```python
from build123d import *

# Parameters (mm, degrees)
EXTRUDE_1_DEPTH        = 35
SKETCH_4_W             = 142
SKETCH_4_H             = 75
CUT_EXTRUDE_2_DEPTH    = 25
SKETCH_5_R             = 29
CUT_EXTRUDE_3_DEPTH    = 11
CHAMFER_3_SIZE         = 3
FILLET_2_R             = 3
SKETCH_7_R             = 3.2
SKETCH_7_R_2           = 3.25
CUT_EXTRUDE_4_DEPTH    = 11
SKETCH_8_R             = 25.025
CUT_EXTRUDE_5_DEPTH    = 11
SKETCH_9_R             = 5.25
CUT_EXTRUDE_6_DEPTH    = 25
HOLE_WIZARD_M6_1_D     = 5
HOLE_WIZARD_M6_1_DEPTH = 15
HOLE_WIZARD_M6_1_TIP   = 1.502151548
HOLE_WIZARD_M5_1_D     = 4.2
SKETCH_17_R            = 32.525
CUT_EXTRUDE_7_DEPTH    = 3


with BuildPart() as part:
    # 草图1 → 凸台-拉伸1 (new body)
    with BuildSketch(Plane.XY):
        Polygon((0, 0), (0, -60), (160, -60), (160, 35), (68, 35), (0, 35), align=None)
    extrude(amount=EXTRUDE_1_DEPTH)

    # 草图4 → 切除-拉伸2 (cut)
    with BuildSketch(Plane(origin=(0, 0, 0), x_dir=(-1, 0, 0), z_dir=(0, 0, -1))):
        with Locations((-77, -12.5)):
            Rectangle(SKETCH_4_W, SKETCH_4_H)
    extrude(amount=-CUT_EXTRUDE_2_DEPTH, mode=Mode.SUBTRACT)

    # 草图5 → 切除-拉伸3 (cut, through all)
    with BuildSketch(Plane(origin=(0, 0, 25), x_dir=(-1, 0, 0), z_dir=(0, 0, -1))):
        with Locations((-113, -19.25)):
            Circle(SKETCH_5_R)
    extrude(amount=-CUT_EXTRUDE_3_DEPTH, mode=Mode.SUBTRACT)

    # 倒角3
    chamfer_3_edges = [part.edges().sort_by_distance(p)[0] for p in [
        (0, 35, 17.5),
        (160, 35, 17.5),
        (160, -60, 17.5),
        (0, -60, 17.5),
    ]]
    chamfer(chamfer_3_edges, length=CHAMFER_3_SIZE)

    # 圆角2
    fillet_2_edges = [part.edges().sort_by_distance(p)[0] for p in [
        (6, 25, 12.5),
        (6, -50, 12.5),
        (148, -50, 12.5),
        (148, 25, 12.5),
    ]]
    fillet(fillet_2_edges, radius=FILLET_2_R)

    # 草图7 → 切除-拉伸4 (cut, through all)
    with BuildSketch(Plane(origin=(0, 0, 25), x_dir=(-1, 0, 0), z_dir=(0, 0, -1))):
        with Locations((-73, -19.25)):
            Circle(SKETCH_7_R)
        with Locations((-141.284271247, -47.534271247)):
            Circle(SKETCH_7_R)
        with Locations((-141.284271247, 9.034271247)):
            Circle(SKETCH_7_R)
        with Locations((-100.534490363, 18.758039538)):
            Circle(SKETCH_7_R_2)
        with Locations((-90.025808003, -51.994259071)):
            Circle(SKETCH_7_R_2)
    extrude(amount=-CUT_EXTRUDE_4_DEPTH, mode=Mode.SUBTRACT)

    # 草图8 → 切除-拉伸5 (cut, through all)
    with BuildSketch(Plane(origin=(0, 0, 25), x_dir=(-1, 0, 0), z_dir=(0, 0, -1))):
        with Locations((-35, -9.275)):
            Circle(SKETCH_8_R)
    extrude(amount=-CUT_EXTRUDE_5_DEPTH, mode=Mode.SUBTRACT)

    # 草图9 → 切除-拉伸6 (cut)
    with BuildSketch(Plane(origin=(0, 0, 0), x_dir=(-1, 0, 0), z_dir=(0, 0, -1))):
        with Locations((-141.284271247, -47.534271247)):
            Circle(SKETCH_9_R)
        with Locations((-90.025808003, -51.994259071)):
            Circle(SKETCH_9_R)
    extrude(amount=-CUT_EXTRUDE_6_DEPTH, mode=Mode.SUBTRACT)

    # M6 螺纹孔1
    with Locations(Plane(origin=(0, 0, 0), x_dir=(-1, 0, 0), z_dir=(0, 0, -1))):
        with Locations((-154, 29), (-80, 29), (-6, 29), (-154, -54), (-6, -54), (-65, -54)):
            Hole(HOLE_WIZARD_M6_1_D / 2, depth=HOLE_WIZARD_M6_1_DEPTH)
            with Locations((0, 0, -(HOLE_WIZARD_M6_1_DEPTH + HOLE_WIZARD_M6_1_TIP / 2))):  # 118° drill point
                Cone(0, HOLE_WIZARD_M6_1_D / 2, HOLE_WIZARD_M6_1_TIP, mode=Mode.SUBTRACT)

    # M5 螺纹孔1 (through all)
    with Locations(Plane.XY.offset(35)):
        with Locations((10.251262658, 15.473737342), (59.748737342, 15.473737342), (59.748737342, -34.023737342), (10.251262658, -34.023737342)):
            Hole(HOLE_WIZARD_M5_1_D / 2)

    # 草图17 → 切除-拉伸7 (cut)
    with BuildSketch(Plane.XY.offset(35)):
        with Locations((113, -19.25)):
            Circle(SKETCH_17_R)
    extrude(amount=-CUT_EXTRUDE_7_DEPTH, mode=Mode.SUBTRACT)


solid = part.part
```
Here's how the part is built. I have some questions about the finished solid (model axes, mm). A direction names the side the tool comes from. Coordinates: 2 decimals unless noted, no trailing zeros. Loops run counter-clockwise (first coordinate to the right, second up) from the corner with the lowest first, then second, coordinate; pieces in that order, holes last. Notation, with made-up numbers: (-7.75, 24.25) -> (48.25, 24.25) arc R21 cw to (48.25, 60.25) -> close; hole circle Ø1 at (64, 86.5). An arc over 180 degrees is marked (long way). Return JSON: item names as keys, results as strings.
1) If we section it at D-D, the plane x = 91: Write out the boundary of the cut face in (y, z).
Results below:
{"outline": "(-60, 0) -> (-57.15, 0) -> (-57.15, 25) -> (-55.09, 25) -> (-55.09, 35) -> (-60, 35) -> close; (-48.89, 25) -> (-38.14, 25) -> (-38.14, 32) -> (-43.21, 32) -> (-43.21, 35) -> (-48.89, 35) -> close; (-0.36, 25) -> (25, 25) -> (25, 0) -> (35, 0) -> (35, 35) -> (4.71, 35) -> (4.71, 32) -> (-0.36, 32) -> close"}
2) Thinking about a two-plate mould opening in X: for faces 1 (the face through (73.694, -22.374, 29.93)), 2 (the face through (79, -60, 17)), 3 (the face through (0, -12, 17)), 4 (the face through (158, 34, 17)), which applies, +X half, -X half, draft (parallel to the pull), parting line (faces both ways), or undercut?
Results below:
{"face 1": "undercut", "face 2": "draft", "face 3": "-X half", "face 4": "+X half"}
3) If we section it at B-B, the plane x = 73: Write out the boundary of the cut face in (y, z), then the cut area to 3 significant figures.
Results below:
{"outline": "(-60, 0) -> (-50, 0) -> (-50, 25) -> (-22.45, 25) -> (-22.45, 35) -> (-60, 35) -> close; (-16.05, 25) -> (25, 25) -> (25, 0) -> (35, 0) -> (35, 35) -> (-16.05, 35) -> close", "area": "1,390 mm²"}
4) If we section it at A-A, the plane z = 3.5: Write out the boundary of the cut face in (x, y).
Results below:
{"outline": "(0, -57) -> (3, -60) -> (157, -60) -> (160, -57) -> (160, 32) -> (157, 35) -> (3, 35) -> (0, 32) -> close; hole circle Ø5 at (6, -54); hole circle Ø5 at (6, 29); hole (6, -47) arc R3 ccw to (9, -50) -> (85.17, -50) arc R5.25 ccw (long way) to (94.88, -50) -> (136.65, -50) arc R5.25 ccw to (146.01, -49.83) arc R3 ccw to (148, -47) -> (148, 22) arc R3 ccw to (145, 25) -> (9, 25) arc R3 ccw to (6, 22) -> close; hole circle Ø5 at (65, -54); hole circle Ø5 at (80, 29); hole circle Ø5 at (154, -54); hole circle Ø5 at (154, 29)"}
5) Will these pins go through, and if not, where does the flat tip stop? pin 1 (10 mm diameter, centred on x = 67, y = -12.5, fed in from -Z); pin 2 (4 mm diameter, centred on x = 154, y = 29, fed in from -Z).
Results below:
{"pin 1": "z = 25", "pin 2": "z = 15.3"}
6) I need wall thicknesses on line 1 (Y direction, x = 65, z = 4); line 2 (Y direction, x = 38, z = 3); line 3 (X direction, y = -26.5, z = 8). Which ranges of each line are inside material? Lowest first, please. Write a range as from..to.
Results below:
{"line 1": "-60..-56.5, -51.5..-50, 25..35", "line 2": "-60..-50, 25..35", "line 3": "0..6, 148..160"}
7) For faces 5 (the face through (8.385, -53.249, 7.605)), 6 (the face through (10.707, -36.074, 29.93)), 7 (the face through (80.506, -17.82, 33.521)), which set-ups out of +Z, -Z, +X, -X, +Y, -Y let a thin tool reach every point of the face, with its end or its side?
Results below:
{"face 5": "-Z", "face 6": "+Z, -Z", "face 7": "+Z"}
8) If we section it at C-C, the plane y = -19.25: Write out the boundary of the cut face in (x, z) (3 decimals).
Results below:
{"outline": "(0, 0) -> (6, 0) -> (6, 25) -> (12.049, 25) -> (12.049, 35) -> (0, 35) -> close; (57.951, 25) -> (69.8, 25) -> (69.8, 35) -> (57.951, 35) -> close; (76.2, 25) -> (84, 25) -> (84, 32) -> (80.475, 32) -> (80.475, 35) -> (76.2, 35) -> close; (142, 25) -> (148, 25) -> (148, 0) -> (160, 0) -> (160, 35) -> (145.525, 35) -> (145.525, 32) -> (142, 32) -> close"}
